Print and shaded views of the part. All mm, measured from the part's lowest x, y and z. Give positions to 0.01 mm unless a question says otherwise; leave off trailing zeros. Loops run counter-clockwise (first coordinate to the right, second up) from the corner with the lowest first, then second, coordinate; pieces in that order, holes last. Notation, with made-up numbers: M 64.5,44.25 L 74.5,44.25 A8 ccw 74.5,54.25 Z; hole C 52,-9.5 d11. An arc over 180 degrees is marked long. Put each result on its own line as item: value. Start each with the question number.
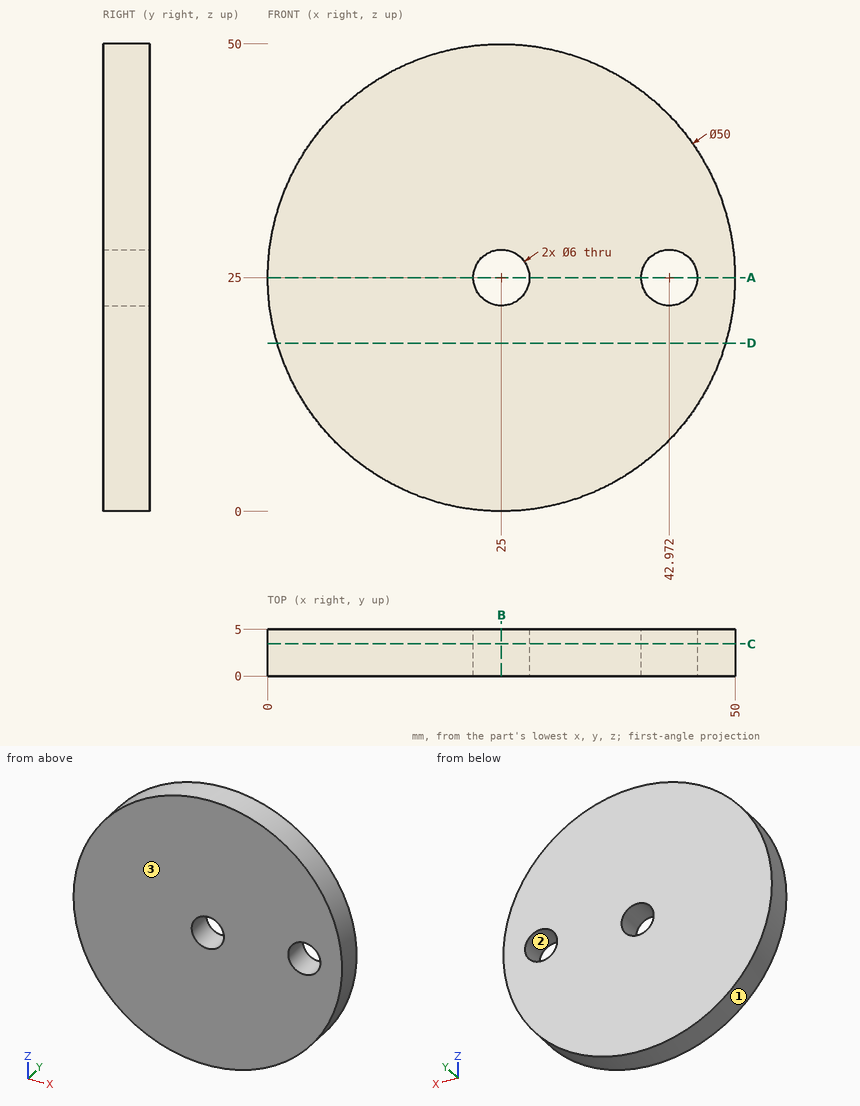
1) Pin check, flat tips, straight feed: pin 1 Ø3 at (y, z) = (4.5, 34) entering from -X; pin 2 Ø2 at (x, y) = (43, 2.5) entering from +Z; pin 3 Ø1.5 at (x, y) = (15, 4) entering from +Z. Stop position of each tip, or through.
2) Mould opens along Z. For the marked faces 1, 2 and 3 say: +Z half, -Z half, draft (parallel to the pull), parting line (faces both ways), or undercut.
3) Wall check: L1, parallel to X at y = 1.7, z = 23 (1 decimal); L2, parallel to Z at x = 25, y = 3.9; L3, parallel to X at y = 2.4, z = 26.5 (1 decimal). Give the ranges that are in metal, low to high.
4) Band-saw the part on A-A on z = 25. Give the cut face in (x, y), then the cut area to 3 significant figures.
5) Band-saw the part on C-C on y = 3.45. Give the cut face in (x, z), then the cut area to 3 significant figures.
6) Band-saw the part on D-D on z = 18. Give the cut face in (x, y), then the cut area to 3 significant figures.
7) Band-saw the part on B-B on x = 25. Give the cut face in (y, z), then the cut area to 3 significant figures.
Evaluation:
1. pin 1: x = 1.15
1. pin 2: z = 43.33
1. pin 3: z = 48.23
2. face 1: parting line
2. face 2: undercut
2. face 3: draft
3. L1: 0.1 to 22.8, 27.2 to 40.7, 45.2 to 49.9
3. L2: 0 to 22, 28 to 50
3. L3: 0 to 22.4, 27.6 to 40.4, 45.6 to 50
4. outline: M 0,0 L 22,0 L 22,5 L 0,5 Z; M 28,0 L 39.97,0 L 39.97,5 L 28,5 Z; M 45.97,0 L 50,0 L 50,5 L 45.97,5 Z
4. area: 190 mm2
5. outline: C 25,25 d50; hole C 25,25 d6; hole C 42.97,25 d6
5. area: 1,910 mm2
6. outline: M 1,0 L 49,0 L 49,5 L 1,5 Z
6. area: 240 mm2
7. outline: M 0,0 L 5,0 L 5,22 L 0,22 Z; M 0,28 L 5,28 L 5,50 L 0,50 Z
7. area: 220 mm2
